The listing builds one solid part. Answer for the finished solid, in the listing's coordinates (mm). A direction names the side the tool comes from. Give positions to 0.01 mm unless a question says otherwise; leave off trailing zeros. Write each loop counter-clockwise with the first axis right and the second up, starting at its lowest first coordinate (ties: lowest second). Pieces come first, ordered by that corner, then holes. Notation, with made-up numbers: (17.5, 17.25) -> (43.5, 17.25) arc R18 cw to (43.5, 43.25) -> close; hole circle Ø5 at (61, 71). An arc over 180 degrees is marked (long way). One line per question, with ' | ' between items.
from build123d import *

# Parameters (mm, degrees)
SKETCH1_W           = 32.7
SKETCH1_H           = 16.35
SKETCH1_R           = 3.175
BOSS_EXTRUDE1_DEPTH = 10
SKETCH2_W           = 5
SKETCH2_H           = 16.35
CUT_EXTRUDE1_DEPTH  = 5


with BuildPart() as part:
    # Sketch1 → Boss-Extrude1 (new, symmetric)
    with BuildSketch(Plane.XY):
        Rectangle(SKETCH1_W, SKETCH1_H)
        with Locations((-8.175, 0)):
            Circle(SKETCH1_R, mode=Mode.SUBTRACT)
        with Locations((8.175, 0)):
            Circle(SKETCH1_R, mode=Mode.SUBTRACT)
    extrude(amount=BOSS_EXTRUDE1_DEPTH, both=True)

    # Sketch2 → Cut-Extrude1 (cut)
    with BuildSketch(Plane(origin=(0, 0, -10), x_dir=(-1, 0, 0), z_dir=(0, 0, -1))):
        with Locations((-8.175, 0)):
            Rectangle(SKETCH2_W, SKETCH2_H)
        with Locations((8.175, 0)):
            Rectangle(SKETCH2_W, SKETCH2_H)
    extrude(amount=-CUT_EXTRUDE1_DEPTH, mode=Mode.SUBTRACT)


solid = part.part
Item 1: A tool of negligible diameter and unlimited length cuts with its end or side. For faces 4 (the face through (-5.675, 5, -8)), 5 (the face through (-8.86, -3.1, -0.14)), from which of +Z, -Z, +X, -X, +Y, -Y can it reach the whole face along a straight path? Write none if from no direction.
Answers below:
face 4: -Z, +Y, -Y | face 5: +Z, -Z
Item 2: A flat-ended cylindrical pin translates along its axis: pin 1 (1.5 mm diameter, centred on x = -7, y = 5.5, fed in from -Z). Find the tip coordinate at first contact, or state that the pin passes through.
Answers below:
pin 1: z = -5
Item 3: Find section B-B (z = -5.5). Write down the section's boundary in (x, y) (3 decimals), then the cut area to 3 significant figures.
Answers below:
outline: (-16.35, -8.175) -> (-10.675, -8.175) -> (-10.675, -1.957) arc R3.175 cw to (-10.675, 1.957) -> (-10.675, 8.175) -> (-16.35, 8.175) -> close; (-5.675, -8.175) -> (5.675, -8.175) -> (5.675, -1.957) arc R3.175 cw to (5.675, 1.957) -> (5.675, 8.175) -> (-5.675, 8.175) -> (-5.675, 1.957) arc R3.175 cw to (-5.675, -1.957) -> close; (10.675, -8.175) -> (16.35, -8.175) -> (16.35, 8.175) -> (10.675, 8.175) -> (10.675, 1.957) arc R3.175 cw to (10.675, -1.957) -> close | area: 364 mm²
Item 4: Determine the mould class of faces 1 (the face through (0, -8.175, 0)), 2 (the face through (-16.35, 0, 0)), 3 (the face through (8, -6, -5)) for opening direction X: pulls with the +X half, pulls with the -X half, needs draft (parallel to the pull), parting line crosses it, or undercut.
Answers below:
face 1: needs draft | face 2: pulls with the -X half | face 3: undercut
Item 5: Find section C-C (x = 7.5). Write down the section's boundary in (y, z) (3 decimals), then the cut area to 3 significant figures.
Answers below:
outline: (-8.175, -5) -> (-3.102, -5) -> (-3.102, 10) -> (-8.175, 10) -> close; (3.102, -5) -> (8.175, -5) -> (8.175, 10) -> (3.102, 10) -> close | area: 152 mm²
Item 6: Consider line 1 (X direction, y = 0, z = 6.25); line 2 (X direction, y = 5.5, z = -8) (3 decimals); line 3 (Y direction, x = -6, z = -0.5) (3 decimals). Determine where each line is inside the solid, lowest interval first. Write a range as [from, to].
Answers below:
line 1: [-16.35, -11.35], [-5, 5], [11.35, 16.35] | line 2: [-16.35, -10.675], [-5.675, 5.675], [10.675, 16.35] | line 3: [-8.175, -2.313], [2.313, 8.175]
Item 7: Find section D-D (z = 2.75). Write down the section's boundary in (x, y) (3 decimals).
Answers below:
outline: (-16.35, -8.175) -> (16.35, -8.175) -> (16.35, 8.175) -> (-16.35, 8.175) -> close; hole circle Ø6.35 at (-8.175, 0); hole circle Ø6.35 at (8.175, 0)
Item 8: Find section A-A (y = 0). Write down the section's boundary in (x, z), then the cut area to 3 significant figures.
Answers below:
outline: (-16.35, -10) -> (-11.35, -10) -> (-11.35, 10) -> (-16.35, 10) -> close; (-5, -10) -> (5, -10) -> (5, 10) -> (-5, 10) -> close; (11.35, -10) -> (16.35, -10) -> (16.35, 10) -> (11.35, 10) -> close | area: 400 mm²
